Check sheet for the modelled part. Datum: model origin and axes. Units: mm. Coordinates: 2 decimals unless noted, no trailing zeros. Loops run counter-clockwise (first coordinate to the right, second up) from the corner with the lowest first, then second, coordinate; pieces in that order, holes last. Notation, with made-up numbers: (27.5, -6) -> (58.5, -6) arc R13 ccw to (58.5, 2) -> close; hole circle Ø4 at (29, -14). An arc over 180 degrees is marked (long way). Use CSV: the item, a comma, the result in double quotes.
Autodesk Inventor part; units mm, degrees
ref_plane "YZ Plane" through (0, 0, 0) normal (1, 0, 0) x (0, 1, 0)
ref_plane "XZ Plane" through (0, 0, 0) normal (0, 1, 0) x (-1, 0, 0)
ref_plane "XY Plane" through (0, 0, 0) normal (0, 0, 1) x (1, 0, 0)
sketch "Эскиз1" plane through (0, 0, 0) normal (1, 0, 0) x (0, 1, 0)
  circle A0 centre (25.7199, 46.7921) radius 2.25
  circle A1 centre (25.6987, 6.5017) radius 4.6
  circle A2 centre (7.6987, 6.5017) radius 1.6
  arc A3 (27.6873, 0.2956) -> (32.7199, 5.2955) centre (27.7199, 5.2955) ccw
  circle A4 centre (7.6843, 30.491) radius 14
  arc A5 (14.2267, 42.8683) -> (-1.4853, 19.9118) centre (7.6843, 30.491) ccw
  circle A6 centre (27.6987, 30.491) radius 1.6
  line L0 (7.6843, 30.491) -> (25.6987, 6.5017)
  line L1 (-6.3157, 30.491) -> (21.6843, 30.491)
  line L2 (7.6843, 16.491) -> (7.6843, 44.491)
  circle A7 centre (7.6843, 30.491) radius 2.5
  circle A8 centre (-0.3157, 30.491) radius 1.6
  circle A9 centre (15.6843, 30.491) radius 1.6
  circle A10 centre (7.6843, 20.991) radius 1.6
  circle A11 centre (7.6843, 39.991) radius 1.6
  circle A12 centre (2.6987, 49.5017) radius 1.5
  circle A13 centre (7.6987, 6.5017) radius 3
  line L3 (7.6987, 3.5017) -> (27.6873, 0.2956)
  circle A14 centre (2.6987, 49.5017) radius 3
  line L4 (-3.2958, 40.9198) -> (-5.3755, 35.5348)
  line L5 (-0.0999, 50.5825) -> (-5.3755, 35.5348)
  line L6 (-1.3769, 17.8835) -> (-4.5981, 23.7723)
  line L7 (-4.5981, 23.7723) -> (5.0667, 5.062)
  circle A15 centre (25.7199, 46.7921) radius 4
  line L8 (2.4504, 52.4914) -> (23, 51)
  line L9 (2.4504, 52.4914) -> (26.0094, 50.7816)
  line L10 (32.7199, 5.2955) -> (29.7095, 47.0795)
  point P0 (0, 0)
  point P1 (-2.3427, 0)
  point P2 (7.6843, 30.491)
  point P3 (7.6843, 30.491)
  point P4 (-4.5981, 23.7723)
  point P5 (-3.3371, 41.4181)
  point P6 (-5.3755, 35.5348)
  point P7 (5.0013, 5.1886)
  point P8 (-0.1621, 50.405)
  point P9 (3.376, 52.4242)
  dimension "d9" = 4.5
  dimension "d86" = 9.2
  dimension "d87" = 3.2
  dimension "d92" = 5
  dimension "d132" = 28
  dimension "d145" = 3.2
  dimension "d191" = 30
  dimension "d194" = 5
  dimension "d195" = 3.2
  dimension "d196" = 3.2
  dimension "d197" = 3.2
  dimension "d198" = 3.2
  dimension "d199" = 8
  dimension "d200" = 8
  dimension "d201" = 9.5
  dimension "d202" = 9.5
  dimension "d227" = 3
  dimension "d234" = 6
  dimension "d235" = 6
  dimension "d242" = 8
extrude "Выдавливание1" add sketch "Эскиз1" along normal blind 2.5 contours A13 | A4 L5 A14 L8 L9 A15 L10 A3 L3 A13 L7 | A4 L2 A10 A7 L0 | L0 A7 L1 A9 A4 | A4 L1 A8 A7 L2 A10 | L1 A9 A7 L2 A11 A4 | L8 A14 | L2 A11 A7 L1 A8 A4 | A15
sketch "Эскиз8" plane through (2.5, 0, 0) normal (1, 0, 0) x (0, 0, -1)
  circle A0 centre (-40.5072, 7.6405) radius 1.6
  circle A1 centre (-40.5072, 7.6405) radius 2.6
  circle A2 centre (-30.9442, -0.3839) radius 1.6
  circle A3 centre (-30.9442, -0.3839) radius 2.6
  circle A4 centre (-21.5765, 7.6255) radius 1.6
  circle A5 centre (-21.5765, 7.6255) radius 2.6
  circle A6 centre (-30.9442, 15.6084) radius 1.6
  circle A7 centre (-30.9442, 15.6084) radius 2.6
  point P0 (0, 0)
  dimension "d205" = 3.2
  dimension "d206" = 5.2
  dimension "d207" = 3.2
  dimension "d208" = 5.2
  dimension "d210" = 3.2
  dimension "d211" = 5.2
  dimension "d216" = 3.2
  dimension "d217" = 5.2
extrude "Выдавливание9" cut sketch "Эскиз8" against normal blind 1.5 contours A0 | A1 | A2 | A3 | A4 | A5 | A6 | A7
equation "\"Радиус_гибки\" = Толщина"
equation "\"Ширина_просечки\" = Толщина"
equation "\"Глубина_просечки\" = 0.5 * Толщина"
equation "\"Размер_просечки\" = 4 * Толщина"
equation "\"Мин_остаток\" = 2 * Толщина"
equation "\"Радиус_перехода\" = Радиус_гибки"
equation "\"Радиус_Якоби\" = Радиус_гибки"
equation "\"Размер_зазора\" = Толщина"
properties part number "drib_rig"
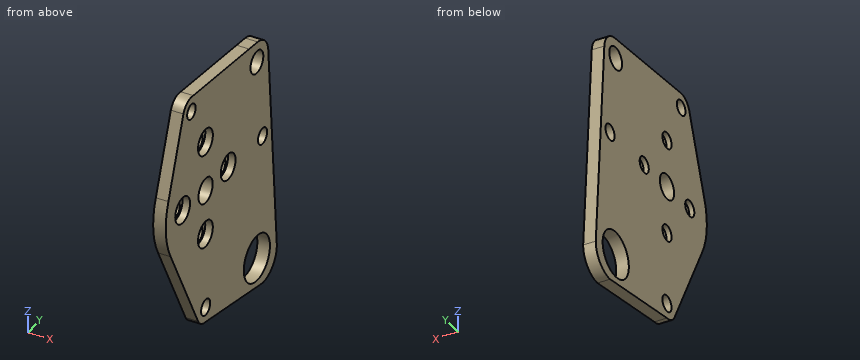
1) Cross-section at D-D on z = 12. Record the boundary of the cut face in (x, y), and give its area (3 significant figures).
Answer below:
outline,"(0, 1.48) -> (2.5, 1.48) -> (2.5, 32.24) -> (0, 32.24) -> close"
area,"76.9 mm²"
2) Cross-section at C-C on y = 20. Record the boundary of the cut face in (x, z).
Answer below:
outline,"(0, 1.53) -> (2.5, 1.53) -> (2.5, 51.22) -> (0, 51.22) -> close"
3) Cross-section at B-B on x = 0.6. Give the number of separate pieces and of enclosed holes in the cut face, and give its area (3 significant figures).
Answer below:
separate pieces,"1"
enclosed holes,"10"
area,"1,470 mm²"
4) Go/stop test with flat-tipped pins: pin 1 Ø3 at (y, z) = (27.7, 30.49) entering from +X; pin 2 Ø1 at (x, y) = (2, 15) entering from +Z; pin 3 Ø1 at (x, y) = (1.5, 18.5) entering from -Z; pin 4 Ø1.5 at (x, y) = (1, 25) entering from -Z. Record where each tip stops, or that it passes through.
Answer below:
pin 1,"passes through"
pin 2,"stops at z = 51.62"
pin 3,"stops at z = 1.69"
pin 4,"stops at z = 0.61"
5) Cross-section at A-A on z = 20. Record the boundary of the cut face in (x, y), and give its area (3 significant figures).
Answer below:
outline,"(0, -2.65) -> (2.5, -2.65) -> (2.5, 5.56) -> (1, 5.56) -> (1, 6.43) -> (0, 6.43) -> close; (0, 8.94) -> (1, 8.94) -> (1, 9.69) -> (2.5, 9.69) -> (2.5, 31.66) -> (0, 31.66) -> close"
area,"77.1 mm²"
6) Thickness scan on line 1 along Z through (x, y) = (2, 1.5); line 2 along Z through (x, y) = (1.25, 5.5); line 3 along Z through (x, y) = (1.3, 9.5). Record the ranges inside material, lowest first. Write a range as from..to.
Answer below:
line 1,"z = 11.97..29.15, 32.74..48.6, 50.4..52.25"
line 2,"z = 4.46..20.08, 23.07..29.27, 31.71..39.03, 41.98..52.27"
line 3,"z = 3.21..19.77, 23.38..28.77, 32.21..38.69, 42.32..51.98"
